from build123d import *

# Parameters (mm, degrees)
SKETCH1_W           = 431.8
SKETCH1_H           = 355.6
BOSS_EXTRUDE1_DEPTH = 0.9906
SKETCH2_W           = 34
SKETCH2_H           = 34
CUT_EXTRUDE1_DEPTH  = 280.690241675
SKETCH3_R           = 16.811779192
SKETCH3_R_2         = 17.94039836
SKETCH3_R_3         = 15.918471064
BOSS_EXTRUDE2_DEPTH = 7.62


with BuildPart() as part:
    # Sketch1 → Boss-Extrude1 (new body)
    with BuildSketch(Plane.XY):
        Rectangle(SKETCH1_W, SKETCH1_H)
    extrude(amount=BOSS_EXTRUDE1_DEPTH)

    # Sketch2 → Cut-Extrude1 (cut, through all)
    with BuildSketch(Plane.XY.offset(0.9906)):
        with Locations((-134.9, -71.3)):
            Rectangle(SKETCH2_W, SKETCH2_H)
    extrude(amount=-CUT_EXTRUDE1_DEPTH, mode=Mode.SUBTRACT)

    # Sketch3 → Boss-Extrude2 (add)
    with BuildSketch(Plane(origin=(0, 0, 0), x_dir=(-1, 0, 0), z_dir=(0, 0, -1))):
        with Locations(Location((-152.604411187, 148.581420283, 0), (0, 0, 180))):
            Circle(SKETCH3_R)
        with Locations(Location((178.932328772, 148.581420283, 0), (0, 0, 180))):
            Circle(SKETCH3_R_2)
        with Locations(Location((-176.007004595, -138.100348975, 0), (0, 0, 180))):
            Circle(SKETCH3_R)
        with Locations(Location((178.932328772, -142.488335239, 0), (0, 0, 180))):
            Circle(SKETCH3_R_3)
    extrude(amount=BOSS_EXTRUDE2_DEPTH)


solid = part.part
Here's how the part is built. I have some questions about the finished solid (model axes, mm). A direction names the side the tool comes from. Give positions to 0.01 mm unless a question says otherwise; leave off trailing zeros. Order: outer loops, then holes, each group sorted by start corner. A loop starts at its lowest first (then second) coordinate and runs counter-clockwise, first axis right, second up. Notation, with made-up numbers: (83.25, -11) -> (104.25, -11) arc R20 ccw to (104.25, 26) -> close; hole circle Ø9 at (16, 87). An arc over 180 degrees is marked (long way). Use a Markdown table: item, result. Add a question column.
Item 1: I need wall thicknesses on line 1 (Z direction, x = -53, y = -132); line 2 (X direction, y = -130.5, z = -1.75); line 3 (X direction, y = -141.5, z = -7). Which ranges of each line are inside material? Lowest first, please.
Item 2: Imagine slicing it at A-A on x = -122.5. Please give me the cut outline in (y, z), plus the area to 3 significant figures.
Item 3: For faces 3 (the face through (-196.855, 147.793, -3.757)), 4 (the face through (-179, 148, -7.62)), which set-ups out of +Z, -Z, +X, -X, +Y, -Y let a thin tool reach every point of the face, with its end or its side?
Item 4: Imagine slicing it at D-D on x = -42. Please give me the cut outline in (y, z).
Item 5: If we mould it in two halves opening along X, with no side actions, what happens to faces 1 (the face through (-191.565, -132.802, -3.757)), 2 (the face through (-179, -143, -7.62))? For each: pulls with the +X half, pulls with the -X half, needs draft (parallel to the pull), parting line crosses it, or undercut.
Item 6: Imagine slicing it at C-C on y = -48. Please give me the cut outline in (x, z).
Item 7: Imagine slicing it at B-B on z = -2.75. Please give me the cut outline in (x, y), plus the area to 3 significant figures.
Data:
| question | item | result |
|---|---|---|
| 1 | line 1 | z = 0 to 0.99 |
| 1 | line 2 | x = -189.41 to -168.46, 161.01 to 191 |
| 1 | line 3 | x = -194.82 to -163.04, 159.54 to 192.47 |
| 2 | outline | (-177.8, 0) -> (-88.3, 0) -> (-88.3, 0.99) -> (-177.8, 0.99) -> close; (-54.3, 0) -> (177.8, 0) -> (177.8, 0.99) -> (-54.3, 0.99) -> close |
| 2 | area | 319 mm² |
| 3 | face 3 | -Z |
| 3 | face 4 | -Z, +X, -X, +Y, -Y |
| 4 | outline | (-177.8, 0) -> (177.8, 0) -> (177.8, 0.99) -> (-177.8, 0.99) -> close |
| 5 | face 1 | undercut |
| 5 | face 2 | needs draft |
| 6 | outline | (-215.9, 0) -> (215.9, 0) -> (215.9, 0.99) -> (-215.9, 0.99) -> close |
| 7 | outline | circle Ø35.88 at (-178.93, 148.58); circle Ø31.84 at (-178.93, -142.49); circle Ø33.62 at (152.6, 148.58); circle Ø33.62 at (176.01, -138.1) |
| 7 | area | 3,580 mm² |
